Solid Edge part; units mm, degrees
sketch "Sketch1" plane through (0, 0, 0) normal (0, -1, 0) x (1, 0, 0)
  circle A0 centre (0, 0) radius 15
extrude "Protrusion1" add sketch "Sketch1" against normal blind 7
sketch "Sketch2" plane through (0, 7, 0) normal (0, 1, 0) x (-1, 0, 0)
  circle A0 centre (0, 0) radius 12.5
extrude "ExtrudedCutout_3" cut sketch "Sketch2" against normal blind 5
chamfer "Chamfer_9" distance 10 distance2 5 1 edges at (12.5, 2, 0) measured on face at (-8.0833, 2, -8.5833)
sketch "Sketch3" plane through (0, 0, 0) normal (0, -1, 0) x (1, 0, 0)
  circle A0 centre (0, 0) radius 7.5
extrude "ExtrudedProtrusion_3" add sketch "Sketch3" along normal blind 3
fillet "Round_2" radius 2 2 edges at (12.5, 7, 0) (-15, 7, 0)
fillet "Round_3" radius 0.5 1 edges at (0, 2, 2.5)
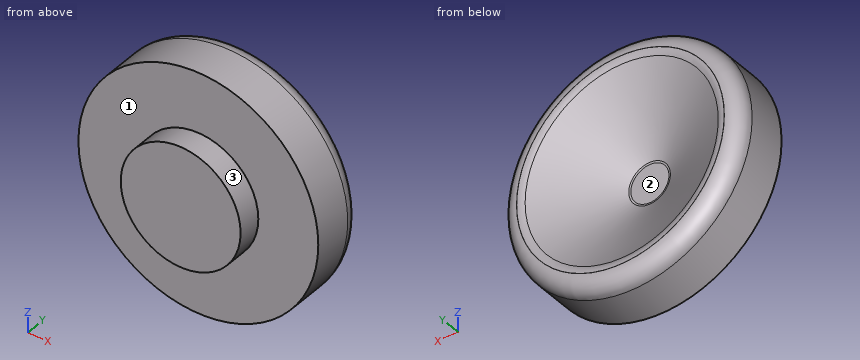
Geometry check sheet. Reference: the model listing, model coordinates, mm. Face numbers are marked on the shaded views. Coordinates: 2 decimals unless noted, no trailing zeros. Loops run counter-clockwise (first coordinate to the right, second up) from the corner with the lowest first, then second, coordinate; pieces in that order, holes last. Notation, with made-up numbers: (62.25, -23) - (95.25, -23) arc R24 cw to (95.25, 3) - close; hole circle Ø9 at (-23, 8). An arc over 180 degrees is marked (long way). One line per item, written item: value. Start each with the question number.
(1) Cross-section at C-C on y = -0.5. Enter the section's corners in (x, z), plus the area to 3 significant figures.
(2) Mould release check, pull along Z, two halves, no side actions. Record for the marked faces 1, 2 and 3: released by +Z, released by -Z, zero draft, split by the parting line, or undercut.
(3) Depth check by flat-ended pin: P1, Ø2, axis at x = 8.5, y = 3, coming from the +Z side; P2, Ø5, axis at x = 0.5, z = -0.5, coming from the +Y side; P3, Ø5, axis at x = -5, y = 1.5, coming from the +Z side. Enter the tip coordinate at first touch or a pass-through.
(4) Material ranges on line 1 (Y direction, x = -11, z = 7); line 2 (X direction, y = 5.5, z = 5.5); line 3 (Z direction, x = 1, y = 3.75), recorded low to high. Write a range as [from, to].
(5) Cross-section at D-D on y = 6. Enter the section's corners in (x, z), plus the area to 3 significant figures.
Results below:
1. outline: circle Ø15 at (0, 0)
1. area: 177 mm2
2. face 1: zero draft
2. face 2: undercut
2. face 3: split by the parting line
3. P1: stops at z = 12.99
3. P2: stops at y = 2.35
3. P3: stops at z = 14.79
4. line 1: y = [0, 7]
4. line 2: x = [-13.89, -7.75], [7.75, 13.89]
4. line 3: z = [-14.97, -5.92], [5.92, 14.97]
5. outline: circle Ø29.46 at (0, 0); hole circle Ø21 at (0, 0)
5. area: 335 mm2
